The figure shows three views and two pictorial views of one solid part (mm, origin at its lowest corner). Answer the questions. A direction names the side the tool comes from. Coordinates: 2 decimals unless noted, no trailing zeros. Loops run counter-clockwise (first coordinate to the right, second up) from the corner with the lowest first, then second, coordinate; pieces in that order, holes last.
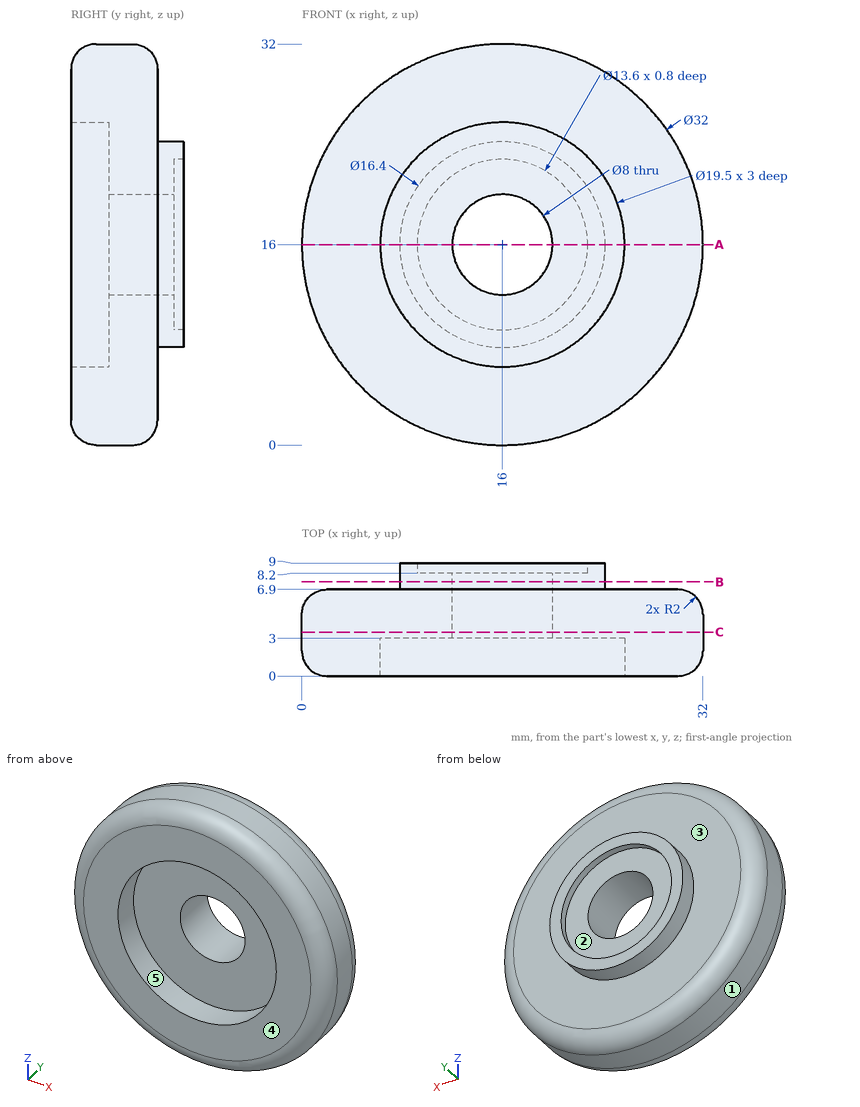
Q1. Which of the six approach directions +Z, -Z, +X, -X, +Y, -Y give full straight-line access (tool end or side, diameter ignored) to the marked faces 4 and 5?
Findings below:
face 4: +Z, -Z, +X, -X, -Y
face 5: -Y
Q2. A cutting plane is placed at A-A (z = 16). Give the vertices of the cut face in (x, y).
Findings below:
outline: (0, 2) arc R2 ccw to (2, 0) - (6.25, 0) - (6.25, 3) - (12, 3) - (12, 8.2) - (9.2, 8.2) - (9.2, 9) - (7.8, 9) - (7.8, 6.9) - (2, 6.9) arc R2 ccw to (0, 4.9) - close; (20, 3) - (25.75, 3) - (25.75, 0) - (30, 0) arc R2 ccw to (32, 2) - (32, 4.9) arc R2 ccw to (30, 6.9) - (24.2, 6.9) - (24.2, 9) - (22.8, 9) - (22.8, 8.2) - (20, 8.2) - close
Q3. Straight lines are drawn through the part: probe 1 along Z at (x, y) = (16, 4.9); probe 2 along Z at (x, y) = (16, 8.7); probe 3 along Y at (x, z) = (3.5, 19). For each, find the intervals that lie inside material, in ascending order.
Findings below:
probe 1: z = 0 to 12, 20 to 32
probe 2: z = 7.8 to 9.2, 22.8 to 24.2
probe 3: y = 0 to 6.9
Q4. A cutting plane is placed at B-B (y = 7.5). Give the vertices of the cut face in (x, z), then the cut area to 3 significant figures.
Findings below:
outline: circle Ø16.4 at (16, 16); hole circle Ø8 at (16, 16)
area: 161 mm2
Q5. Flat-ended cylindrical pins translate along their axes: pin 1 Ø10.5 at (x, z) = (16, 16) entering from -Y; pin 2 Ø6 at (x, z) = (3.5, 15) entering from +Y; pin 3 Ø11.5 at (x, z) = (16, 16) entering from +Y. Find the tip coordinate at first contact, or state that the pin passes through.
Findings below:
pin 1: stops at y = 3
pin 2: stops at y = 6.9
pin 3: stops at y = 8.2
Q6. A cutting plane is placed at C-C (y = 3.5). Give the vertices of the cut face in (x, z), then the cut area to 3 significant figures.
Findings below:
outline: circle Ø32 at (16, 16); hole circle Ø8 at (16, 16)
area: 754 mm2
Q7. Determine the mould class of the marked faces 1, 2 and 3 for opening direction X: +X half, -X half, draft (parallel to the pull), parting line (faces both ways), or undercut.
Findings below:
face 1: parting line
face 2: undercut
face 3: draft
